Verification items for the finished model (mm, model axes). Coordinates: 2 decimals unless noted, no trailing zeros. Write each loop counter-clockwise with the first axis right and the second up, starting at its lowest first coordinate (ties: lowest second). Pieces come first, ordered by that corner, then holes. Notation, with made-up numbers: (0, 34) -> (40, 34) arc R24 cw to (40, 71) -> close; hole circle Ø9 at (-36.75, -9.75). An arc over 180 degrees is marked (long way). Answer in a Markdown table with one row per item.
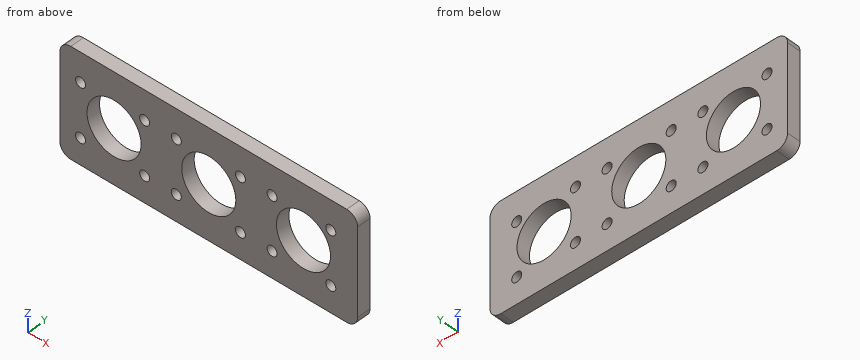
```python
from build123d import *

# Parameters (mm, degrees)
F0_W          = 139.7
F0_H          = 50.8
F0_R          = 12.7
F1_DEPTH      = 6.35
F2_R          = 5.08
F3_R          = 2.3495
F4_DEPTH      = 25.4
F4_DEPTH_BACK = 25.4


with BuildPart() as f1:
    # F0 (on Front) → F1 (new body)
    with BuildSketch(Plane.XZ):
        with Locations((-3.385224, -11.762154)):
            Rectangle(F0_W, F0_H)
        with Locations((-47.835224, -11.762154)):
            Circle(F0_R, mode=Mode.SUBTRACT)
        with Locations((-3.385224, -11.762154)):
            Circle(F0_R, mode=Mode.SUBTRACT)
        with Locations((41.064776, -11.762154)):
            Circle(F0_R, mode=Mode.SUBTRACT)
    extrude(amount=F1_DEPTH)

    # F2
    f2_edges = [f1.edges().sort_by_distance(p)[0] for p in [
        (-73.235224, -3.175, 13.637846),
        (66.464776, -3.175, 13.637846),
        (66.464776, -3.175, -37.162154),
        (-73.235224, -3.175, -37.162154),
    ]]
    fillet(f2_edges, radius=F2_R)

    # F3 (on face) → F4 (cut, two sides)
    with BuildSketch(Plane.XZ.offset(6.35)) as f4_sk:
        with Locations((-63.577805, 0)):
            Circle(F3_R)
        with Locations((-33.478805, 0)):
            Circle(F3_R)
        with Locations((-63.577805, -24.933804)):
            Circle(F3_R)
        with Locations((-33.478805, -24.933804)):
            Circle(F3_R)
        with Locations((-18.619805, 0)):
            Circle(F3_R)
        with Locations((11.479195, 0)):
            Circle(F3_R)
        with Locations((-18.619805, -24.933804)):
            Circle(F3_R)
        with Locations((11.479195, -24.933804)):
            Circle(F3_R)
        with Locations((26.338195, 0)):
            Circle(F3_R)
        with Locations((53.897195, 0)):
            Circle(F3_R)
        with Locations((26.338195, -24.933804)):
            Circle(F3_R)
        with Locations((53.897195, -24.933804)):
            Circle(F3_R)
    extrude(amount=-F4_DEPTH, mode=Mode.SUBTRACT)
    extrude(f4_sk.sketch, amount=-F4_DEPTH_BACK, mode=Mode.SUBTRACT)


solid = f1.part
```
1. Sectioned sample at B-B, the plane x = -6.5. Record the cut outline in (y, z).
Findings below:
| item | result |
|---|---|
| outline | (-6.35, -37.16) -> (0, -37.16) -> (0, -24.07) -> (-6.35, -24.07) -> close; (-6.35, 0.55) -> (0, 0.55) -> (0, 13.64) -> (-6.35, 13.64) -> close |
2. Sectioned sample at D-D, the plane y = -4. Count the separate pieces of the cut face and the enclosed holes in it, and give its area (3 significant figures).
Findings below:
| item | result |
|---|---|
| separate pieces | 1 |
| enclosed holes | 15 |
| area | 5,350 mm² |
3. Sectioned sample at A-A, the plane x = 55. Record the cut outline in (y, z).
Findings below:
| item | result |
|---|---|
| outline | (-6.35, -37.16) -> (0, -37.16) -> (0, -27.01) -> (-6.35, -27.01) -> close; (-6.35, -22.86) -> (0, -22.86) -> (0, -2.07) -> (-6.35, -2.07) -> close; (-6.35, 2.07) -> (0, 2.07) -> (0, 13.64) -> (-6.35, 13.64) -> close |
4. Go/stop test with a flat-tipped pin: pin 1 (4 mm diameter, centred on x = -33.48, z = 0, fed in from -Y). Record where the tip stops, or that it passes through.
Findings below:
| item | result |
|---|---|
| pin 1 | passes through |
5. Sectioned sample at C-C, the plane z = -21. Record the cut outline in (x, y), and give its area (3 significant figures).
Findings below:
| item | result |
|---|---|
| outline | (-73.24, -6.35) -> (-56.55, -6.35) -> (-56.55, 0) -> (-73.24, 0) -> close; (-39.12, -6.35) -> (-12.1, -6.35) -> (-12.1, 0) -> (-39.12, 0) -> close; (5.33, -6.35) -> (32.35, -6.35) -> (32.35, 0) -> (5.33, 0) -> close; (49.78, -6.35) -> (66.46, -6.35) -> (66.46, 0) -> (49.78, 0) -> close |
| area | 555 mm² |
6. Material ranges on probe 1 along X at (y, z) = (-6, -12); probe 2 along Z at (x, y) = (-47.5, -3.75); probe 3 along X at (y, z) = (-2, -5.5), recorded low to high. Write a range as from..to.
Findings below:
| item | result |
|---|---|
| probe 1 | x = -73.24..-60.53, -35.14..-16.08, 9.31..28.37, 53.76..66.46 |
| probe 2 | z = -37.16..-24.46, 0.93..13.64 |
| probe 3 | x = -73.24..-58.88, -36.79..-14.43, 7.66..30.02, 52.11..66.46 |
